from build123d import *

# Parameters (mm, degrees)
SKETCH1_R           = 110
BOSS_EXTRUDE1_DEPTH = 6
SKETCH2_R           = 7.5
CUT_EXTRUDE1_DEPTH  = 156.679157243
CAVITY1_START       = 73.692998072
CAVITY1_OUTLINE_W   = 6
CAVITY1_OUTLINE_H   = 6
CAVITY1_DEPTH       = 6
CUT_EXTRUDE2_DEPTH  = 156.679157243
SKETCH6_R           = 1.5
CUT_EXTRUDE3_DEPTH  = 156.679157243


# Read off the part's stored shape, not the designer's step: Cavity1
with BuildPart() as part:
    # Sketch1 → Boss-Extrude1 (new body)
    with BuildSketch(Plane(origin=(0, 0, 0), x_dir=(1, 0, 0), z_dir=(0, 1, 0))):
        with Locations(Location((0, 0, 0), (0, 0, 270))):
            Circle(SKETCH1_R)
    extrude(amount=BOSS_EXTRUDE1_DEPTH)

    # Sketch2 → Cut-Extrude1 (cut, through all)
    with BuildSketch(Plane(origin=(0, 6, 0), x_dir=(1, 0, 0), z_dir=(0, 1, 0))):
        with Locations(Location((0, 40, 0), (0, 0, 270))):
            Circle(SKETCH2_R)
    extrude(amount=-CUT_EXTRUDE1_DEPTH, mode=Mode.SUBTRACT)

    # Cavity1 outline → Cavity1 (cut)
    with BuildSketch(Plane(origin=(0, 0, 0), x_dir=(0, 1, 0), z_dir=(0.998532697756286, 0, 0.0541521145621647)).offset(CAVITY1_START)):
        with Locations((3, -19.041827)):
            Rectangle(CAVITY1_OUTLINE_W, CAVITY1_OUTLINE_H)
        with Locations((3, 19.958173)):
            Rectangle(CAVITY1_OUTLINE_W, CAVITY1_OUTLINE_H)
    extrude(amount=CAVITY1_DEPTH, mode=Mode.SUBTRACT)

    # Sketch3 → Cut-Extrude2 (cut, through all)
    with BuildSketch(Plane(origin=(0, 6, 0), x_dir=(1, 0, 0), z_dir=(0, 1, 0))):
        Polygon((-21.248834596, -78.65774343), (-20.923921909, -72.666547244), (-26.915118096, -72.341634556), (-27.240030783, -78.332830743), align=None)
        Polygon((17.693940616, -80.769675898), (11.702744429, -80.444763211), (12.027657117, -74.453567024), (18.018853303, -74.778479712), align=None)
        Polygon((-78.65774343, 21.248834596), (-72.666547244, 20.923921909), (-72.341634556, 26.915118096), (-78.332830743, 27.240030783), align=None)
        Polygon((-80.769675898, -17.693940616), (-80.444763211, -11.702744429), (-74.453567024, -12.027657117), (-74.778479712, -18.018853303), align=None)
        Polygon((21.248834596, 78.65774343), (20.923921909, 72.666547244), (26.915118096, 72.341634556), (27.240030783, 78.332830743), align=None)
        Polygon((-17.693940616, 80.769675898), (-11.702744429, 80.444763211), (-12.027657117, 74.453567024), (-18.018853303, 74.778479712), align=None)
    extrude(amount=-CUT_EXTRUDE2_DEPTH, mode=Mode.SUBTRACT)

    # Sketch6 → Cut-Extrude3 (cut, through all)
    with BuildSketch(Plane(origin=(0, 6, 0), x_dir=(1, 0, 0), z_dir=(0, 1, 0))):
        with Locations(Location((0, 90, 0), (0, 0, 270))):
            Circle(SKETCH6_R)
        with Locations(Location((0, 0, 0), (0, 0, 270))):
            Circle(SKETCH6_R)
    extrude(amount=-CUT_EXTRUDE3_DEPTH, mode=Mode.SUBTRACT)


solid = part.part
The listing builds one solid part. Answer for the finished solid, in the listing's coordinates (mm). Give positions to 0.01 mm unless a question says otherwise; leave off trailing zeros. Write each loop counter-clockwise with the first axis right and the second up, starting at its lowest first coordinate (ties: lowest second). Pieces come first, ordered by that corner, then holes. Notation, with made-up numbers: (-14.75, -32.75) -> (41.25, -32.75) arc R7 ccw to (41.25, -22.75) -> close; hole circle Ø7 at (89.5, 52.25). An arc over 180 degrees is marked (long way). One line per question, with ' | ' between items. Start each with the question number.
1. Given pin 1 Ø3 at (x, y) = (-73, 2) entering from -Z; pin 2 Ø3 at (x, y) = (-81, 4.5) entering from +Z; pin 3 Ø2 at (x, y) = (87.5, 2.5) entering from +Z, each flat-ended and moving along its own axis, determine where each tip first touches the part or whether it passes through.
2. Find the intervals of material crossed by probe 1 along X at (y, z) = (1.5, 0); probe 2 along X at (y, z) = (1.9, -40); probe 3 along Z at (x, y) = (-17, 1), in increasing order.
3. Section C-C (x = 51.5) is taken. Determine the outline of the cut face in (y, z).
4. Section A-A (z = -40) is taken. Determine the outline of the cut face in (x, y), plus the area to 3 significant figures.
5. For a pull along X with two mould halves and no side action, classify faces 1 (the flat face through (14.981, 3.042, 74.614)), 2 (the flat face through (2, 6, -2)) as pulls with the +X half, pulls with the -X half, needs draft (parallel to the pull), parting line crosses it, or undercut.
6. Section D-D (z = 69) is taken. Determine the outline of the cut face in (x, y).
7. Section B-B (y = 4) is taken. State how many separate pieces and enclosed holes the cut face has, plus the area to 3 significant figures.
Response values:
1) pin 1: z = -83.59 | pin 2: z = 76.02 | pin 3: z = 67.95
2) probe 1: -110 to -1.5, 1.5 to 110 | probe 2: -102.47 to -7.5, 7.5 to 102.47 | probe 3: -108.68 to -80.73, -74.72 to 108.68
3) outline: (0, -97.2) -> (6, -97.2) -> (6, 97.2) -> (0, 97.2) -> close
4) outline: (-102.47, 0) -> (-7.5, 0) -> (-7.5, 6) -> (-102.47, 6) -> close; (7.5, 0) -> (102.47, 0) -> (102.47, 6) -> (7.5, 6) -> close | area: 1,140 mm2
5) face 1: undercut | face 2: needs draft
6) outline: (-85.67, 0) -> (85.67, 0) -> (85.67, 6) -> (-85.67, 6) -> close
7) separate pieces: 1 | enclosed holes: 11 | area: 37,500 mm2
